from build123d import *

# Parameters (mm, degrees)
F0_W     = 1500
F0_H     = 2000
F0_W_2   = 1400
F0_H_2   = 1900
F1_DEPTH = 470
F2_W     = 20
F2_H     = 450
F3_DEPTH = 450
F5_DEPTH = 450
F6_W     = 470
F6_H     = 20
F7_DEPTH = 450


with BuildPart() as f1:
    # F0 (on Front) → F1 (new body)
    with BuildSketch(Plane.XZ):
        Rectangle(F0_W, F0_H)
        Rectangle(F0_W_2, F0_H_2, mode=Mode.SUBTRACT)
    extrude(amount=F1_DEPTH)

    # F2 (on Front) → F3 (join)
    with BuildSketch(Plane.XZ):
        Polygon((700, -500), (700, -480), (-700, -480), (-700, -500), (-250, -500), (-230, -500), (230, -500), (250, -500), align=None)
        with Locations((240, -725)):
            Rectangle(F2_W, F2_H)
        with Locations((-240, -725)):
            Rectangle(F2_W, F2_H)
    extrude(amount=F3_DEPTH)

    # F4 (on Front) → F5 (join)
    with BuildSketch(Plane.XZ):
        Polygon((230, 950), (210, 950), (210, 500), (-700, 500), (-700, 480), (230, 480), align=None)
    extrude(amount=F5_DEPTH)

    # F6 (on Front) → F7 (join)
    with BuildSketch(Plane.XZ):
        with Locations((465, 490)):
            Rectangle(F6_W, F6_H)
    extrude(amount=F7_DEPTH)


solid = f1.part
Can you work these out from the model? Positions are in its coordinate system, mm. A direction names the side the tool comes from. Give positions to 0.01 mm unless a question says otherwise; leave off trailing zeros. Loops run counter-clockwise (first coordinate to the right, second up) from the corner with the lowest first, then second, coordinate; pieces in that order, holes last. Notation, with made-up numbers: M 60.25,-2 L 105.25,-2 A15 ccw 105.25,6 Z; hole C 61,86.5 d1. An arc over 180 degrees is marked long. One line per item, written item: value.
1) Imagine slicing it at B-B on x = 153. Write out the boundary of the cut face in (y, z), and give its area (3 significant figures).
Geometry check:
outline: M -470,-1000 L 0,-1000 L 0,-950 L -470,-950 Z; M -470,950 L 0,950 L 0,1000 L -470,1000 Z; M -450,-500 L 0,-500 L 0,-480 L -450,-480 Z; M -450,480 L 0,480 L 0,500 L -450,500 Z
area: 65,000 mm²
2) Imagine slicing it at D-D on y = -151. Write out the boundary of the cut face in (x, z).
Geometry check:
outline: M -750,-1000 L 750,-1000 L 750,1000 L -750,1000 Z; hole M -700,-950 L -250,-950 L -250,-500 L -700,-500 Z; hole M -700,-480 L 700,-480 L 700,480 L -700,480 Z; hole M -700,500 L 210,500 L 210,950 L -700,950 Z; hole M -230,-950 L 230,-950 L 230,-500 L -230,-500 Z; hole M 230,500 L 700,500 L 700,950 L 230,950 Z; hole M 250,-950 L 700,-950 L 700,-500 L 250,-500 Z
3) Please list where these lines run through material, in increasing order: line 1 (Z direction, x = -134, y = -257); line 2 (X direction, y = -183, z = 706); line 3 (X direction, y = -161.5, z = -891).
Geometry check:
line 1: z = -1000 to -950, -500 to -480, 480 to 500, 950 to 1000
line 2: x = -750 to -700, 210 to 230, 700 to 750
line 3: x = -750 to -700, -250 to -230, 230 to 250, 700 to 750
4) Imagine slicing it at A-A on z = -809. Write out the boundary of the cut face in (x, y), and give its area (3 significant figures).
Geometry check:
outline: M -750,-470 L -700,-470 L -700,0 L -750,0 Z; M -250,-450 L -230,-450 L -230,0 L -250,0 Z; M 230,-450 L 250,-450 L 250,0 L 230,0 Z; M 700,-470 L 750,-470 L 750,0 L 700,0 Z
area: 65,000 mm²
5) Imagine slicing it at C-C on z = -151. Write out the boundary of the cut face in (x, y).
Geometry check:
outline: M -750,-470 L -700,-470 L -700,0 L -750,0 Z; M 700,-470 L 750,-470 L 750,0 L 700,0 Z
6) On a 3-axis mill with a long thin cutter (end or side, diameter ignored), from which of +Z, -Z, +X, -X, +Y, -Y can I reach the whole of each face in a straight line? I mean faces 4 (the face through (472, -222, -500)), 5 (the face through (-3, -450, -488)), 6 (the face through (-726, -470, 5)). Say none if no direction works.
Geometry check:
face 4: +Y, -Y
face 5: -Y
face 6: +Z, -Z, +X, -X, -Y
7) Thinking about a two-plate mould opening in Z: for faces 1 (the face through (-10, -232, 1000)), 2 (the face through (750, -232, -14)), 3 (the face through (-3, -450, 490)), which applies, +Z half, -Z half, draft (parallel to the pull), parting line (faces both ways), or undercut?
Geometry check:
face 1: +Z half
face 2: draft
face 3: undercut
